Work out the finished part from the listing and answer in its coordinate system (mm). Round coordinates to 2 decimals unless told otherwise and drop trailing zeros. Write each loop counter-clockwise with the first axis right and the second up, starting at its lowest first coordinate (ties: lowest second). Pieces come first, ordered by that corner, then holes.
Autodesk Inventor part; units mm, degrees
ref_plane "YZ Plane" through (0, 0, 0) normal (1, 0, 0) x (0, 1, 0)
ref_plane "XZ Plane" through (0, 0, 0) normal (0, 1, 0) x (-1, 0, 0)
ref_plane "XY Plane" through (0, 0, 0) normal (0, 0, 1) x (1, 0, 0)
sketch "Szkic1" plane through (0, 0, 0) normal (0, 1, 0) x (-1, 0, 0)
  line L0 (0, 0) -> (80, 0)
  line L1 (80, 0) -> (80, -25)
  line L2 (80, -25) -> (0, -25)
  line L3 (0, -25) -> (0, 0)
  line L4 (80, -12.5) -> (0, -12.5) construction
  circle A0 centre (61.5, -7.5) radius 2.8
  circle A1 centre (61.5, -17.5) radius 2.8
  circle A2 centre (20, -7.5) radius 2.8
  circle A3 centre (20, -17.5) radius 2.8
  line L5 (80, 0) -> (100, 0)
  line L6 (100, 0) -> (100, -25)
  line L7 (100, -25) -> (80, -25)
  line L8 (80, -25) -> (80, 0)
  line L9 (0, 0) -> (-20, 0)
  line L10 (-20, 0) -> (-20, -25)
  line L11 (-20, -25) -> (0, -25)
  line L12 (0, -25) -> (0, 0)
  circle A4 centre (-10, -7.5) radius 2.8
  circle A5 centre (-10, -17.5) radius 2.8
  circle A6 centre (90, -7.5) radius 2.8
  circle A7 centre (90, -17.5) radius 2.8
  dimension "d0" = 80
  dimension "d1" = 25
  dimension "d2" = 5.6
  dimension "d3" = 10
  dimension "d4" = 20
  dimension "d5" = 18.5
  dimension "d6" = 10
  dimension "d9" = 20
  dimension "d10" = 20
  dimension "d12" = 10
  dimension "d13" = 10
  dimension "d14" = 10
  dimension "d15" = 10
extrude "Wyciągnięcie proste1" add sketch "Szkic1" along normal blind 4
fillet "Zaokrąglenie1" radius 2 4 edges at (-100, 2, 0) (20, 2, 0) (20, 2, -25) (-100, 2, -25)
equation "\"d6\" = d3"
equation "\"d13\" = d3"
equation "\"d14\" = 0.5 * d10"
equation "\"d15\" = 0.5 * d9"
properties part number "belka_wzdluz" material "PLA"
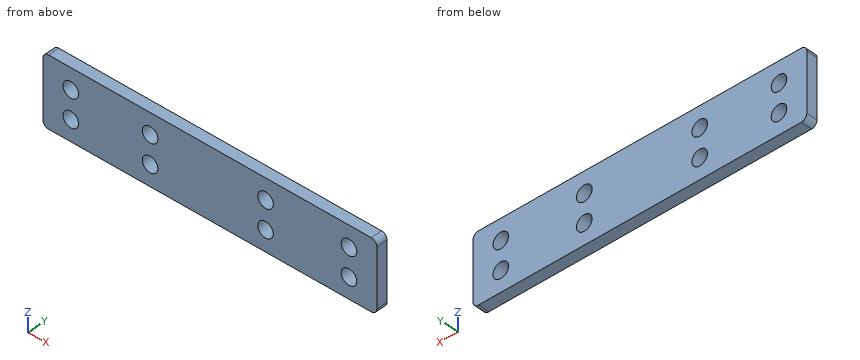
Q1. Find the intervals of material crossed by L1, parallel to X at y = 3, z = -17.25; L2, parallel to Z at x = -61.5, y = 1.9; L3, parallel to X at y = 1.3, z = -8.5, in increasing order.
Q2. Find section C-C (y = 2.4). Count the separate pieces of the cut face and the enclosed holes in it, plus the area to 3 significant figures.
Q3. Find section B-B (x = -20). Determine the outline of the cut face in (y, z), plus the area to 3 significant figures.
Q4. Find section A-A (z = -17.5). Determine the outline of the cut face in (x, y).
Q5. Given pin 1 (3.5 mm diameter, centred on x = -90, z = -7.5, fed in from +Y), flat-ended and moving along its own axis, determine where the tip first touches the part or whether it passes through.
Report:
1. L1: x = -100 to -92.79, -87.21 to -64.29, -58.71 to -22.79, -17.21 to 7.21, 12.79 to 20
1. L2: z = -25 to -20.3, -14.7 to -10.3, -4.7 to 0
1. L3: x = -100 to -92.62, -87.38 to -64.12, -58.88 to -22.62, -17.38 to 7.38, 12.62 to 20
2. separate pieces: 1
2. enclosed holes: 8
2. area: 2,800 mm2
3. outline: (0, -25) - (4, -25) - (4, -20.3) - (0, -20.3) - close; (0, -14.7) - (4, -14.7) - (4, -10.3) - (0, -10.3) - close; (0, -4.7) - (4, -4.7) - (4, 0) - (0, 0) - close
3. area: 55.2 mm2
4. outline: (-100, 0) - (-92.8, 0) - (-92.8, 4) - (-100, 4) - close; (-87.2, 0) - (-64.3, 0) - (-64.3, 4) - (-87.2, 4) - close; (-58.7, 0) - (-22.8, 0) - (-22.8, 4) - (-58.7, 4) - close; (-17.2, 0) - (7.2, 0) - (7.2, 4) - (-17.2, 4) - close; (12.8, 0) - (20, 0) - (20, 4) - (12.8, 4) - close
5. pin 1: passes through
